from build123d import *

# Parameters (mm, degrees)
PAD_DEPTH       = 35
SKETCH001_R     = 27.5
PAD001_DEPTH    = 30
FILLET_R        = 20
THICKNESS_T     = -5
FILLET001_R     = 15
FILLET002_R     = 5
CHAMFER_SIZE2   = 25
CHAMFER_SIZE    = 3
FILLET003_R     = 20
SKETCH002_R     = 28.5
PAD002_DEPTH    = 15
SKETCH003_R     = 25.5
POCKET_DEPTH    = 80.001
SKETCH004_W     = 9
SKETCH004_H     = 20
PAD003_DEPTH    = 5
FILLET004_R     = 7
SKETCH006_R     = 1.5
POCKET002_DEPTH = 40.001
POCKET003_DEPTH = 2.5
POCKET004_DEPTH = 70.001


with BuildPart() as part:
    # Sketch → Pad (new body, symmetric)
    with BuildSketch(Plane.YZ):
        Polygon((-85, 0), (-85, 15), (-35, 65), (35, 65), (35, 0), align=None)
    extrude(amount=PAD_DEPTH, both=True)

    # Sketch001 (on Face2 of Pad) → Pad001 (join)
    with BuildSketch(Plane(origin=(0, -50, 50), x_dir=(0, -0.707107, -0.707107), z_dir=(0, -0.707107, 0.707107))):
        with Locations((14.142136, 0)):
            Circle(SKETCH001_R)
    extrude(amount=PAD001_DEPTH)

    # Fillet
    fillet_edges = [part.edges().sort_by_distance(p)[0] for p in [
        (-35, 35, 32.5),
        (-35, -85, 7.5),
        (35, -85, 7.5),
        (35, 35, 32.5),
    ]]
    fillet(fillet_edges, radius=FILLET_R)

    # Thickness
    thickness_openings = [part.faces().sort_by_distance(p)[0] for p in [
        (0, -25, 0),
        (0, -81.213203, 61.213203),
    ]]
    offset(amount=THICKNESS_T, openings=thickness_openings)

    # Fillet001
    fillet001_edges = [part.edges().sort_by_distance(p)[0] for p in [
        (0, -35, 65),
    ]]
    fillet(fillet001_edges, radius=FILLET001_R)

    # Fillet002
    fillet002_edges = [part.edges().sort_by_distance(p)[0] for p in [
        (-35, -6.893398, 65),
    ]]
    fillet(fillet002_edges, radius=FILLET002_R)

    # Chamfer
    chamfer_edges = [part.edges().sort_by_distance(p)[0] for p in [
        (0, -65.303301, 77.123106),
    ]]
    chamfer_side = part.faces().sort_by_distance((0, -62.317767, 80.10864))[0]
    chamfer(chamfer_edges, length=CHAMFER_SIZE, length2=CHAMFER_SIZE2, reference=chamfer_side)

    # Fillet003
    fillet003_edges = [part.edges().sort_by_distance(p)[0] for p in [
        (-25.606602, 25.606602, 60),
    ]]
    fillet(fillet003_edges, radius=FILLET003_R)

    # Sketch002 (on Face41 of Fillet003) → Pad002 (join)
    with BuildSketch(Plane.XY.offset(65)):
        Circle(SKETCH002_R)
    extrude(amount=PAD002_DEPTH)

    # Sketch003 (on Face46 of Pad002) → Pocket (cut, through all)
    with BuildSketch(Plane.XY.offset(80)):
        Circle(SKETCH003_R)
    extrude(amount=-POCKET_DEPTH, mode=Mode.SUBTRACT)

    # Sketch004 → Pad003 (join, symmetric)
    with BuildSketch(Plane(origin=(0, 0, 0), x_dir=(-1, 0, 0), z_dir=(0, 1, 0))):
        with Locations((-30.5, 70)):
            Rectangle(SKETCH004_W, SKETCH004_H)
        with Locations((30.5, 70)):
            Rectangle(SKETCH004_W, SKETCH004_H)
    extrude(amount=PAD003_DEPTH, both=True)

    # Fillet004
    fillet004_edges = [part.edges().sort_by_distance(p)[0] for p in [
        (35, 0, 80),
        (-35, 0, 80),
    ]]
    fillet(fillet004_edges, radius=FILLET004_R)

    # Sketch006 (on Face2 of Fillet004) → Pocket002 (cut, through all)
    with BuildSketch(Plane.XZ.offset(5)):
        with Locations((-31.528988, 71.49976)):
            Circle(SKETCH006_R)
        with Locations((31.528988, 71.49976)):
            Circle(SKETCH006_R)
    extrude(amount=-POCKET002_DEPTH, mode=Mode.SUBTRACT)

    # Sketch007 (on Face11 of Pocket002) → Pocket003 (cut)
    with BuildSketch(Plane(origin=(0, 5, 0), x_dir=(-1, 0, 0), z_dir=(0, 1, 0))):
        Polygon((-28.778988, 69.912047), (-28.778988, 73.087473), (-31.528988, 74.675186), (-34.278988, 73.087473), (-34.278988, 69.912047), (-31.528988, 68.324333), align=None)
        Polygon((34.278988, 69.912047), (34.278988, 73.087473), (31.528988, 74.675186), (28.778988, 73.087473), (28.778988, 69.912047), (31.528988, 68.324333), align=None)
    extrude(amount=-POCKET003_DEPTH, mode=Mode.SUBTRACT)

    # Sketch008 (on Face16 of Pocket003) → Pocket004 (cut, through all)
    with BuildSketch(Plane(origin=(-35, 0, 0), x_dir=(0, -1, 0), z_dir=(-1, 0, 0))):
        Polygon((0, 94.046894), (120.73246, 94.046894), (120.73246, 0), (8.694593, 0), (8.694593, 7.939231), (4.694593, 7.939231), (4, 4), (0, 4), align=None)
    extrude(amount=-POCKET004_DEPTH, mode=Mode.SUBTRACT)


solid = part.part
CAD build for the part. Positions are in the model's coordinates, mm. A direction names the side the tool comes from. Round coordinates to 2 decimals unless told otherwise and drop trailing zeros. Write each loop counter-clockwise with the first axis right and the second up, starting at its lowest first coordinate (ties: lowest second). Pieces come first, ordered by that corner, then holes.
(1) Slice it at A-A, the plane y = 9. Write the cut outline in (x, z), and give its area (3 significant figures).
(2) Mould opens along X. For faces 4 (the face through (-34, 10, 63)), 5 (the face through (-25.72, 25.49, 19.72)), 6 (the face through (-33, -7, 7.939)) say: pulls with the +X half, pulls with the -X half, needs draft (parallel to the pull), parting line crosses it, or undercut.
(3) Probe line 1 along X through (y, z) = (13, 3); line 2 along Y through (x, z) = (11, 7.5); line 3 along Z through (x, y) = (25.5, 10). List the from-to ranges inside material, lowest first.
(4) Drop flat-ended pins along their axis: P1, Ø4, axis at x = -31.53, z = 71.5, coming from the -Y side; P2, Ø1.2, axis at x = -33, y = -1, coming from the +Z side; P3, Ø6, axis at x = 10, z = 9.5, coming from the -Y side. Give the stop position or say it passes through.
(5) 3-axis set-ups, long thin cutter, end or side, ignore diameter. For faces 1 (the face through (0, 30, 20)), 2 (the face through (-30.17, 3.77, 73.89)), 3 (the face through (-28.4, 5, 72.4)): which of +Z, -Z, +X, -X, +Y, -Y reach the whole face in a straight line?
(6) Slice it at B-B, the plane x = 7. Write the cut outline in (y, z).
From the geometry:
1. outline: (-35, 0) - (-30, 0) - (-30, 40) arc R20 cw to (-23.86, 54.42) - (-23.86, 80) - (-27.04, 80) - (-27.04, 65) - (-30, 65) arc R5 ccw to (-35, 60) - close; (23.86, 54.42) arc R20 cw to (30, 40) - (30, 0) - (35, 0) - (35, 60) arc R5 ccw to (30, 65) - (27.04, 65) - (27.04, 80) - (23.86, 80) - close
1. area: 920 mm2
2. face 4: pulls with the -X half
2. face 5: undercut
2. face 6: needs draft
3. line 1: x = -35 to -30, 30 to 35
3. line 2: y = 30 to 35
3. line 3: z = 52.64 to 80
4. P1: stops at y = 0
4. P2: stops at z = 4
4. P3: stops at y = 30
5. face 1: -Z, -Y
5. face 2: +Y
5. face 3: +Z, -X, +Y
6. outline: (24.52, 53.75) arc R20 cw to (30, 40) - (30, 0) - (35, 0) - (35, 60) arc R5 ccw to (30, 65) - (27.63, 65) - (27.63, 80) - (24.52, 80) - close
